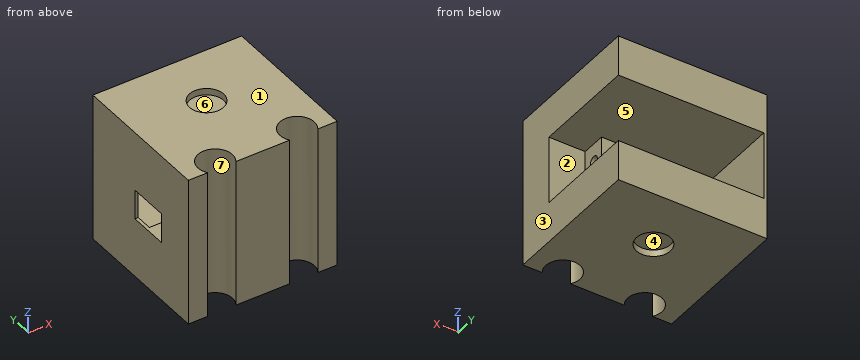
```python
from build123d import *

# Parameters (mm, degrees)
SKETCH1_W                = 45
SKETCH1_H                = 50
BOSS_EXTRUDE1_DEPTH      = 45
SKETCH2_R                = 5.2
CUT_EXTRUDE1_DEPTH       = 45
SKETCH9_R                = 5.15
CUT_EXTRUDE6_DEPTH       = 2
SKETCH10_R               = 5.15
CUT_EXTRUDE7_DEPTH       = 2
SKETCH12_R               = 12.7
CUT_EXTRUDE8_DEPTH       = 46
SKETCH13_W               = 45
SKETCH13_H               = 6.66747138
CUT_EXTRUDE9_DEPTH       = 46
SKETCH16_R               = 13.25
SKETCH16_R_2             = 3.75
BOSS_EXTRUDE3_DEPTH      = 2
SKETCH20_R               = 12.7
BOSS_EXTRUDE4_DEPTH      = 45
SKETCH21_W               = 20.5
SKETCH21_H               = 40.5
CUT_EXTRUDE10_DEPTH      = 44
SKETCH22_R               = 2.15
BOSS_EXTRUDE5_DEPTH      = 44
SKETCH26_W               = 5.127085864
SKETCH26_H               = 8
CUT_EXTRUDE16_DEPTH      = 7
SKETCH28_R               = 2.15
BOSS_EXTRUDE6_DEPTH      = 44
SKETCH29_R               = 2.15
CUT_EXTRUDE18_DEPTH      = 10
SKETCH30_W               = 8
SKETCH30_H               = 7
CUT_EXTRUDE19_DEPTH      = 7
CUT_EXTRUDE19_DEPTH_BACK = 7
SKETCH31_W               = 20.5
SKETCH31_H               = 7.407828578
CUT_EXTRUDE20_DEPTH      = 11
SKETCH32_W               = 9
SKETCH32_H               = 5.046358254
CUT_EXTRUDE21_DEPTH      = 14
SKETCH33_W               = 8.088030226
SKETCH33_H               = 9
CUT_EXTRUDE22_DEPTH      = 7
SKETCH34_R               = 1.6
CUT_EXTRUDE23_DEPTH      = 10
SKETCH35_W               = 5
SKETCH35_H               = 9
CUT_EXTRUDE24_DEPTH      = 7


with BuildPart() as part:
    # Sketch1 → Boss-Extrude1 (new body)
    with BuildSketch(Plane.XY):
        with Locations((8.236607143, -2.901785714)):
            Rectangle(SKETCH1_W, SKETCH1_H)
    extrude(amount=BOSS_EXTRUDE1_DEPTH)

    # Sketch2 → Cut-Extrude1 (cut)
    with BuildSketch(Plane.XY.offset(45)):
        with Locations((-4.163392857, -24.901785714)):
            Circle(SKETCH2_R)
        with Locations((20.636607143, -24.901785714)):
            Circle(SKETCH2_R)
    extrude(amount=-CUT_EXTRUDE1_DEPTH, mode=Mode.SUBTRACT)

    # Sketch9 → Cut-Extrude6 (cut)
    with BuildSketch(Plane.XY.offset(45)):
        with Locations((8.236607143, -2.401785714)):
            Circle(SKETCH9_R)
    extrude(amount=-CUT_EXTRUDE6_DEPTH, mode=Mode.SUBTRACT)

    # Sketch10 → Cut-Extrude7 (cut)
    with BuildSketch(Plane(origin=(0, 0, 0), x_dir=(-1, 0, 0), z_dir=(0, 0, -1))):
        with Locations((-8.236607143, -2.401785714)):
            Circle(SKETCH10_R)
    extrude(amount=-CUT_EXTRUDE7_DEPTH, mode=Mode.SUBTRACT)

    # Sketch12 → Cut-Extrude8 (cut)
    with BuildSketch(Plane.ZY.offset(14.263392857)):
        with Locations((22.5, 0)):
            Circle(SKETCH12_R)
    extrude(amount=-CUT_EXTRUDE8_DEPTH, mode=Mode.SUBTRACT)

    # Sketch13 → Cut-Extrude9 (cut)
    with BuildSketch(Plane.ZY.offset(14.263392857)):
        with Locations((22.5, 18.764478596)):
            Rectangle(SKETCH13_W, SKETCH13_H)
    extrude(amount=-CUT_EXTRUDE9_DEPTH, mode=Mode.SUBTRACT)

    # Sketch16 → Boss-Extrude3 (add)
    with BuildSketch(Plane(origin=(30.736607143, 0, 0), x_dir=(0, 0, -1), z_dir=(1, 0, 0))):
        with Locations((-22.5, 0)):
            Circle(SKETCH16_R)
        with Locations((-22.5, 0)):
            Circle(SKETCH16_R_2, mode=Mode.SUBTRACT)
    extrude(amount=-BOSS_EXTRUDE3_DEPTH)

    # Sketch20 → Boss-Extrude4 (add)
    with BuildSketch(Plane.ZY.offset(14.263392857)):
        with Locations((22.5, 0)):
            Circle(SKETCH20_R)
    extrude(amount=-BOSS_EXTRUDE4_DEPTH)

    # Sketch21 → Cut-Extrude10 (cut)
    with BuildSketch(Plane(origin=(30.736607143, 0, 0), x_dir=(0, 0, -1), z_dir=(1, 0, 0))):
        with Locations((-22.5, 3.75)):
            Rectangle(SKETCH21_W, SKETCH21_H)
    extrude(amount=-CUT_EXTRUDE10_DEPTH, mode=Mode.SUBTRACT)

    # Sketch22 → Boss-Extrude5 (add)
    with BuildSketch(Plane(origin=(30.736607143, 0, 0), x_dir=(0, 0, -1), z_dir=(1, 0, 0))):
        Polygon((-32.5, -8.699027625), (-12.5, -8.699027625), (-12.25, -8.699027625), (-12.25, -16.5), (-32.75, -16.5), (-32.75, -8.699027625), align=None)
        with Locations((-27.215250341, -10.949027625)):
            Circle(SKETCH22_R, mode=Mode.SUBTRACT)
        with Locations((-17.715250341, -10.949027625)):
            Circle(SKETCH22_R, mode=Mode.SUBTRACT)
    extrude(amount=-BOSS_EXTRUDE5_DEPTH)

    # Sketch26 → Cut-Extrude16 (cut)
    with BuildSketch(Plane(origin=(0, -8.699027625, 0), x_dir=(1, 0, 0), z_dir=(0, 1, 0))):
        with Locations((-10.699849925, -22.5)):
            Rectangle(SKETCH26_W, SKETCH26_H)
    extrude(amount=-CUT_EXTRUDE16_DEPTH, mode=Mode.SUBTRACT)

    # Sketch28 → Boss-Extrude6 (add)
    with BuildSketch(Plane(origin=(30.736607143, 0, 0), x_dir=(0, 0, -1), z_dir=(1, 0, 0))):
        with Locations((-27.215250341, -10.949027625)):
            Circle(SKETCH28_R)
        with Locations((-17.715250341, -10.949027625)):
            Circle(SKETCH28_R)
    extrude(amount=-BOSS_EXTRUDE6_DEPTH)

    # Sketch29 → Cut-Extrude18 (cut)
    with BuildSketch(Plane(origin=(30.736607143, 0, 0), x_dir=(0, 0, -1), z_dir=(1, 0, 0))):
        with Locations((-27.215250341, -12.199027625)):
            Circle(SKETCH29_R)
        with Locations((-17.715250341, -12.199027625)):
            Circle(SKETCH29_R)
    extrude(amount=-CUT_EXTRUDE18_DEPTH, mode=Mode.SUBTRACT)

    # Sketch30 → Cut-Extrude19 (cut, two sides)
    with BuildSketch(Plane(origin=(-13.263392857, 0, 0), x_dir=(0, 0, -1), z_dir=(1, 0, 0))) as cut_extrude19_sk:
        with Locations((-22.5, -12.199027625)):
            Rectangle(SKETCH30_W, SKETCH30_H)
    extrude(amount=CUT_EXTRUDE19_DEPTH, mode=Mode.SUBTRACT)
    extrude(cut_extrude19_sk.sketch, amount=-CUT_EXTRUDE19_DEPTH_BACK, mode=Mode.SUBTRACT)

    # Sketch31 → Cut-Extrude20 (cut)
    with BuildSketch(Plane(origin=(30.736607143, 0, 0), x_dir=(0, 0, -1), z_dir=(1, 0, 0))):
        with Locations((-22.5, -12.402941914)):
            Rectangle(SKETCH31_W, SKETCH31_H)
    extrude(amount=-CUT_EXTRUDE20_DEPTH, mode=Mode.SUBTRACT)

    # Sketch32 → Cut-Extrude21 (cut)
    with BuildSketch(Plane(origin=(-13.263392857, 0, 0), x_dir=(0, 0, -1), z_dir=(1, 0, 0))):
        with Locations((-22.5, -6.175848498)):
            Rectangle(SKETCH32_W, SKETCH32_H)
    extrude(amount=-CUT_EXTRUDE21_DEPTH, mode=Mode.SUBTRACT)

    # Sketch33 → Cut-Extrude22 (cut)
    with BuildSketch(Plane(origin=(0, -8.699027625, 0), x_dir=(1, 0, 0), z_dir=(0, 1, 0))):
        with Locations((-10.219377744, -22.5)):
            Rectangle(SKETCH33_W, SKETCH33_H)
    extrude(amount=-CUT_EXTRUDE22_DEPTH, mode=Mode.SUBTRACT)

    # Sketch34 → Cut-Extrude23 (cut)
    with BuildSketch(Plane(origin=(19.736607143, 0, 0), x_dir=(0, 0, -1), z_dir=(1, 0, 0))):
        with Locations((-27.215250341, -12.199027625)):
            Circle(SKETCH34_R)
        with Locations((-17.715250341, -12.199027625)):
            Circle(SKETCH34_R)
    extrude(amount=-CUT_EXTRUDE23_DEPTH, mode=Mode.SUBTRACT)

    # Sketch35 → Cut-Extrude24 (cut)
    with BuildSketch(Plane(origin=(0, -8.699027625, 0), x_dir=(1, 0, 0), z_dir=(0, 1, 0))):
        with Locations((-3.675362631, -22.5)):
            Rectangle(SKETCH35_W, SKETCH35_H)
    extrude(amount=-CUT_EXTRUDE24_DEPTH, mode=Mode.SUBTRACT)


solid = part.part
```
Geometry: final body of the model. Coordinates: model frame, mm. Face numbers are marked on the shaded views. A direction names the side the tool comes from. Coordinates: 2 decimals unless noted, no trailing zeros. Order: outer loops, then holes, each group sorted by start corner. A loop starts at its lowest first (then second) coordinate and runs counter-clockwise, first axis right, second up. Notation, with made-up numbers: (-7, -5.5) -> (29, -5.5) arc R21 cw to (29, 7.5) -> close; hole circle Ø2 at (65.25, 20.5). An arc over 180 degrees is marked (long way). Write each question's results on one line, items separated by ' | '. Start each with the question number.
1) Material intervals for line 1 along Z through (x, y) = (-10, 8); line 2 along Z through (x, y) = (8.5, 0); line 3 along X through (y, z) = (-22.5, 34), sorted ascending.
2) Cut plane D-D, the plane z = 42. Output: boundary loops of the cut face in (x, y), and give its area (3 significant figures).
3) First-contact query: pin 1 (10 mm diameter, centred on x = 18.5, z = 17.5, fed in from +Y); pin 2 (8 mm diameter, centred on x = 8.24, y = -2.4, fed in from +Z); pin 3 (5 mm diameter, centred on y = -12.2, z = 17.72, fed in from +X). Flat tips, straight axial feed; report the tip coordinate or a pass-through.
4) Mould query, pull axis Z, two halves, no side actions, for the marked faces 1, 2, 3 and 4. Classes: released by +Z, released by -Z, zero draft, split by the parting line, or undercut.
5) Cut plane C-C, the plane y = 6. Output: boundary loops of the cut face in (x, z).
6) Cut plane A-A, the plane y = -21.5. Output: boundary loops of the cut face in (x, z), and give its area (3 significant figures).
7) Cut plane B-B, the plane x = -11. Output: boundary loops of the cut face in (y, z).
8) Set-up query: the marked faces 5, 6 and 7. Return all of +Z, -Z, +X, -X, +Y, -Y with unobstructed straight access to the full face (end or side cutting, diameter ignored); none if empty.
Checks:
1) line 1: 0 to 12.25, 32.75 to 45 | line 2: 2 to 12.25, 32.75 to 43 | line 3: -14.26 to -8.78, 0.45 to 16.02, 25.25 to 30.74
2) outline: (-14.26, -27.9) -> (-8.41, -27.9) arc R5.2 cw (long way) to (0.08, -27.9) -> (16.39, -27.9) arc R5.2 cw (long way) to (24.88, -27.9) -> (30.74, -27.9) -> (30.74, 15.43) -> (-14.26, 15.43) -> close | area: 1,810 mm^2
3) pin 1: y = -8.7 | pin 2: z = 43 | pin 3: x = 19.74
4) face 1: released by +Z | face 2: undercut | face 3: zero draft | face 4: released by -Z
5) outline: (-14.26, 0) -> (30.74, 0) -> (30.74, 12.25) -> (-13.26, 12.25) -> (-13.26, 32.75) -> (30.74, 32.75) -> (30.74, 45) -> (-14.26, 45) -> close
6) outline: (-14.26, 0) -> (-8.1, 0) -> (-8.1, 45) -> (-14.26, 45) -> close; (-0.23, 0) -> (16.7, 0) -> (16.7, 45) -> (-0.23, 45) -> close; (24.57, 0) -> (30.74, 0) -> (30.74, 45) -> (24.57, 45) -> close | area: 1,320 mm^2
7) outline: (-27.9, 0) -> (15.43, 0) -> (15.43, 12.25) -> (-8.7, 12.25) -> (-8.7, 18) -> (-15.7, 18) -> (-15.7, 27) -> (-8.7, 27) -> (-8.7, 32.75) -> (15.43, 32.75) -> (15.43, 45) -> (-27.9, 45) -> close
8) face 5: +X, +Y | face 6: +Z | face 7: +Z, -Z
